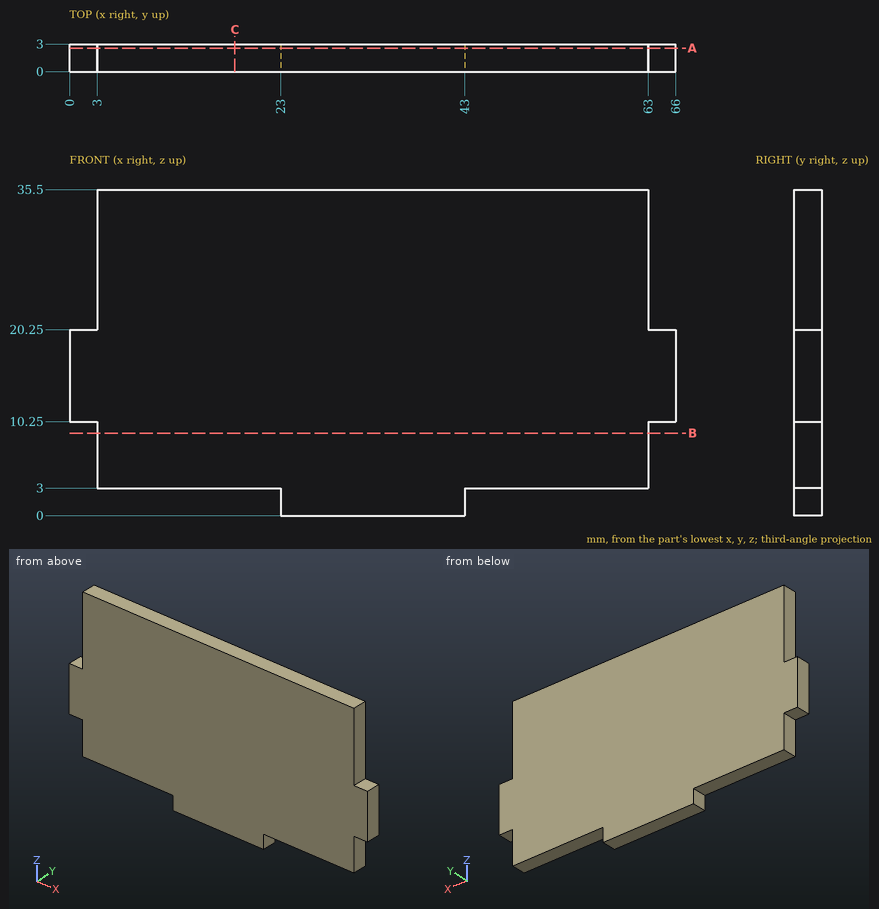
Study the drawing (mm; zero at the part's minimum x, y, z) and answer. Give positions to 0.01 mm unless a question says otherwise; leave off trailing zeros. Loops run counter-clockwise (first coordinate to the right, second up) from the corner with the lowest first, then second, coordinate; pieces in that order, holes last. Notation, with made-up numbers: (-33.5, 38) -> (-16.5, 38) arc R25 ccw to (-16.5, 76) -> close; hole circle Ø3 at (24, -26). An arc over 180 degrees is marked (long way). Use a Markdown table: item, result. Add a question column.
1) The part is cut by section B-B, the plane z = 9. Determine the outline of the cut face in (x, y).
2) Each of these flat-tipped pins is pushed along its axis until it touches: P1, Ø1.5, axis at y = 1, z = 1.5, coming from the -X side; P2, Ø0.9, axis at x = 10, y = 1, coming from the -Z side; P3, Ø0.9, axis at x = 64, y = 1, coming from the -Z side. Where does it stop, or does it pass through?
3) Consider line 1 along X through (y, z) = (1.6, 33.5); line 2 along Z through (x, y) = (51, 1.6); line 3 along X through (y, z) = (0.95, 1). Determine where each line is inside the solid, lowest interval first.
4) The part is cut by section A-A, the plane y = 2.55. Determine the outline of the cut face in (x, z), plus the area to 3 significant figures.
5) The part is cut by section C-C, the plane x = 18. Determine the outline of the cut face in (y, z), plus the area to 3 significant figures.
Reported:
| question | item | result |
|---|---|---|
| 1 | outline | (3, 0) -> (63, 0) -> (63, 3) -> (3, 3) -> close |
| 2 | P1 | stops at x = 23 |
| 2 | P2 | stops at z = 3 |
| 2 | P3 | stops at z = 10.25 |
| 3 | line 1 | x = 3 to 63 |
| 3 | line 2 | z = 3 to 35.5 |
| 3 | line 3 | x = 23 to 43 |
| 4 | outline | (0, 10.25) -> (3, 10.25) -> (3, 3) -> (23, 3) -> (23, 0) -> (43, 0) -> (43, 3) -> (63, 3) -> (63, 10.25) -> (66, 10.25) -> (66, 20.25) -> (63, 20.25) -> (63, 35.5) -> (3, 35.5) -> (3, 20.25) -> (0, 20.25) -> close |
| 4 | area | 2,070 mm^2 |
| 5 | outline | (0, 3) -> (3, 3) -> (3, 35.5) -> (0, 35.5) -> close |
| 5 | area | 97.5 mm^2 |
